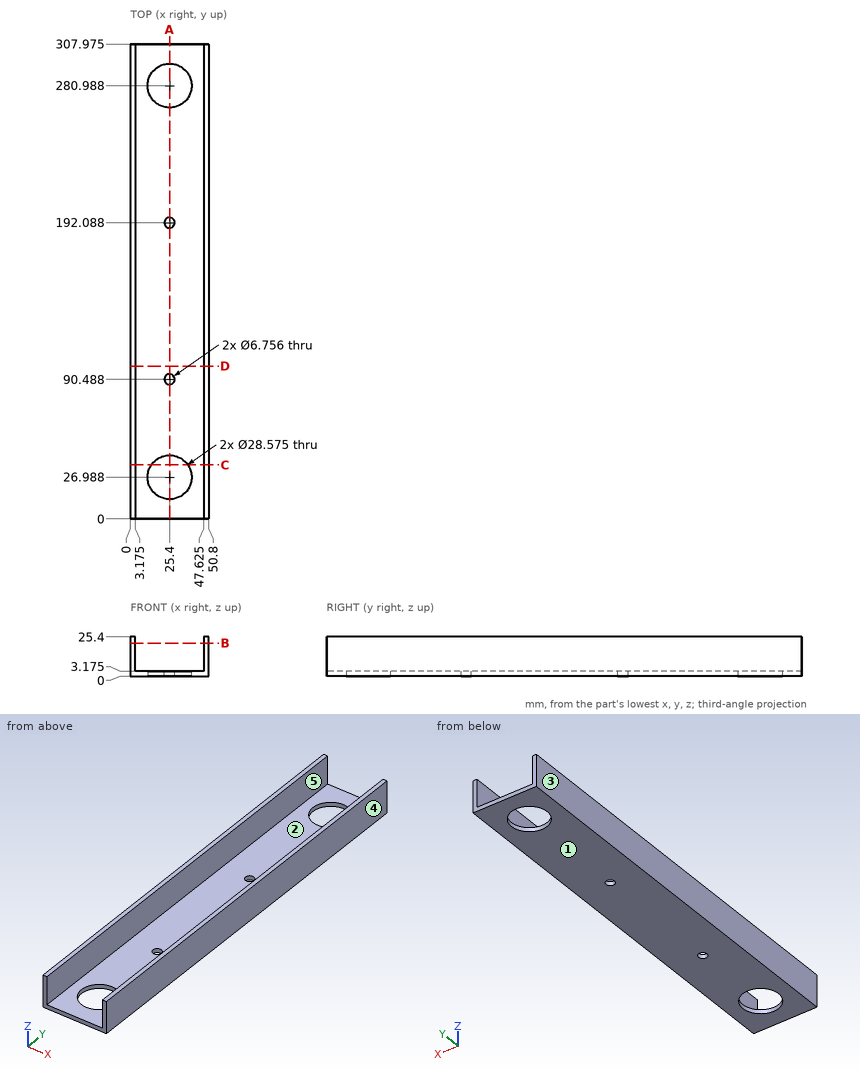
Can you work these out from the drawing? Everything is in mm from the part's minimum corner. A direction names the side the tool comes from. Round coordinates to 2 decimals unless told otherwise and drop trailing zeros. Loops run counter-clockwise (first coordinate to the right, second up) from the corner with the lowest first, then second, coordinate; pieces in that order, holes last. Notation, with made-up numbers: (83.5, -5) -> (136.5, -5) arc R29 ccw to (136.5, 28) -> close; hole circle Ø3 at (75, 46.5). An arc over 180 degrees is marked (long way). Put each result on its own line as item: value.
Q1. I want a section at D-D on y = 99. Write out the boundary of the cut face in (x, z) (1 decimal).
Checks:
outline: (0, 0) -> (50.8, 0) -> (50.8, 25.4) -> (47.6, 25.4) -> (47.6, 3.2) -> (3.2, 3.2) -> (3.2, 25.4) -> (0, 25.4) -> close
Q2. For pin 1 Ø11 at (x, y) = (25.4, 90.49) entering from +Z (1 decimal); pin 2 Ø23 at (x, y) = (25.4, 280.99) entering from -Z, each with a flat end and sliding along its axis, tell me the tip position at first contact or that it passes through.
Checks:
pin 1: z = 3.2
pin 2: through
Q3. Which directions (+Z, -Z, +X, -X, +Y, -Y) give clear straight access to the entire face, cutting with the end or side of a thin tool? Please do the marked faces 4 and 5.
Checks:
face 4: +Z, -Z, +X, +Y, -Y
face 5: +Z, +Y, -Y
Q4. Please list where these lines run through material, in increasing order: line 1 (Y direction, x = 25.4, z = 0.75) (1 decimal); line 2 (X direction, y = 240.5, z = 5.5) (1 decimal); line 3 (Z direction, x = 27, y = 258) (1 decimal). Write a range as from..to.
Checks:
line 1: 0..12.7, 41.3..87.1, 93.9..188.7, 195.5..266.7, 295.3..308
line 2: 0..3.2, 47.6..50.8
line 3: 0..3.2
Q5. Thinking about a two-plate mould opening in X: for the marked faces 1, 2 and 3, which applies, pulls with the +X half, pulls with the -X half, needs draft (parallel to the pull), parting line crosses it, or undercut?
Checks:
face 1: needs draft
face 2: undercut
face 3: pulls with the -X half
Q6. I want a section at B-B on z = 21.25. Write out the boundary of the cut face in (x, y) (1 decimal).
Checks:
outline: (0, 0) -> (3.2, 0) -> (3.2, 308) -> (0, 308) -> close; (47.6, 0) -> (50.8, 0) -> (50.8, 308) -> (47.6, 308) -> close
Q7. I want a section at C-C on y = 35. Write out the boundary of the cut face in (x, z) (1 decimal).
Checks:
outline: (0, 0) -> (13.6, 0) -> (13.6, 3.2) -> (3.2, 3.2) -> (3.2, 25.4) -> (0, 25.4) -> close; (37.2, 0) -> (50.8, 0) -> (50.8, 25.4) -> (47.6, 25.4) -> (47.6, 3.2) -> (37.2, 3.2) -> close
Q8. I want a section at A-A on x = 25.4. Write out the boundary of the cut face in (y, z) (1 decimal).
Checks:
outline: (0, 0) -> (12.7, 0) -> (12.7, 3.2) -> (0, 3.2) -> close; (41.3, 0) -> (87.1, 0) -> (87.1, 3.2) -> (41.3, 3.2) -> close; (93.9, 0) -> (188.7, 0) -> (188.7, 3.2) -> (93.9, 3.2) -> close; (195.5, 0) -> (266.7, 0) -> (266.7, 3.2) -> (195.5, 3.2) -> close; (295.3, 0) -> (308, 0) -> (308, 3.2) -> (295.3, 3.2) -> close
